Verification items for the finished model (mm, model axes). A direction names the side the tool comes from. Coordinates: 2 decimals unless noted, no trailing zeros. Order: outer loops, then holes, each group sorted by start corner. A loop starts at its lowest first (then second) coordinate and runs counter-clockwise, first axis right, second up.
Q1. Thickness scan on line 1 (Z direction, x = 0.75, y = 0.75); line 2 (X direction, y = 4.5, z = -1); line 3 (X direction, y = 3.75, z = 1.5). Record the ranges inside material, lowest first.
Q2. Cross-section at B-B, the plane y = 7.5. Record the boundary of the cut face in (x, z).
Q3. Set-up check for faces 1 (the flat face through (2, 11, 1.242)), 2 (the flat face through (-1.621, 10.034, -1.7)), 3 (the conical face through (-2.409, -2.189, 1.847)), 4 (the cylindrical face through (-0.9, 8.3, -2.1)), 5 (the conical face through (-1.913, 9.933, 0.04)): record each of +Z, -Z, +X, -X, +Y, -Y from which the full face is reachable in a straight line by a thin tool's end or side.
Q4. Draft check along Z on faces 6 (the flat face through (1.194, 9.5, 1.8)), 7 (the flat face through (-2, 11, -1.242)), 8 (the cylindrical face through (0.679, -2.129, -2.156)). Enter one of: pulls with the +Z half, pulls with the -Z half, needs draft (parallel to the pull), parting line crosses it, or undercut.
Q5. Cross-section at C-C, the plane y = 0.75. Record the boundary of the cut face in (x, z), and give its area (3 significant figures).
Q6. Depth check by flat-ended pin: P1, Ø1.5, axis at x = 0.5, z = 0.5, coming from the +Y side; P2, Ø0.7, axis at y = 9.5, z = 2, coming from the -X side; P3, Ø1, axis at x = 2, y = 11, coming from the +Z side. Enter the tip coordinate at first touch or a pass-through.
Q7. Cross-section at A-A, the plane y = -2. Record the boundary of the cut face in (x, z).
from build123d import *

# Parameters (mm, degrees)
SKETCH1_R                   = 2.9972
INSERT_DEPTH                = 11.811
INSERT_TAPER                = 2
INSERT_OTHER_WAY_DEPTH      = 4.318
INSERT_OTHER_WAY_TAPER      = -1
SKETCH2_R                   = 2.2606
INSERT_BORE_DEPTH           = 13.584955674
INSERT_BORE_TAPER           = 2
INSERT_BORE_OTHER_WAY_DEPTH = 13.584955674
PASS_CUT_DEPTH              = 13.584955674
PASS_CUT_DEPTH_BACK         = 13.584955674
PASS_CHIP_DEPTH             = 13.584955674
CIRPATTERN1_COUNT           = 2
SKETCH5_R                   = 2.032
BOSS_EXTRUDE1_DEPTH         = 1.0922


with BuildPart() as part:
    # Sketch1 → insert (new body)
    with BuildSketch(Plane(origin=(0, 0, 0), x_dir=(1, 0, 0), z_dir=(0, 1, 0))):
        Circle(SKETCH1_R)
    extrude(amount=INSERT_DEPTH, taper=INSERT_TAPER)

    # Sketch1 → insert other way (add)
    with BuildSketch(Plane(origin=(0, 0, 0), x_dir=(1, 0, 0), z_dir=(0, 1, 0))):
        Circle(SKETCH1_R)
    extrude(amount=-INSERT_OTHER_WAY_DEPTH, taper=INSERT_OTHER_WAY_TAPER)

    # Sketch2 → insert bore (cut)
    with BuildSketch(Plane.XZ):
        with Locations(Location((0, 0, 0), (0, 0, 270))):
            Circle(SKETCH2_R)
    extrude(amount=-INSERT_BORE_DEPTH, taper=INSERT_BORE_TAPER, mode=Mode.SUBTRACT)

    # Sketch2 → insert bore other way (cut)
    with BuildSketch(Plane.XZ):
        with Locations(Location((0, 0, 0), (0, 0, 270))):
            Circle(SKETCH2_R)
    extrude(amount=INSERT_BORE_OTHER_WAY_DEPTH, mode=Mode.SUBTRACT)

    # Sketch3 → pass cut (cut, two sides: drawn at the far end of the back side and taken through both)
    with BuildSketch(Plane.XY.offset(-PASS_CUT_DEPTH_BACK)):
        with BuildLine():
            Line((-1.1938, 11.811), (1.1938, 11.811))
            Line((1.1938, 11.811), (1.1938, 9.017))
            ThreePointArc((1.1938, 9.017), (0.89622049, 8.29857951), (0.1778, 8.001))
            Line((0.1778, 8.001), (-0.1778, 8.001))
            ThreePointArc((-0.1778, 8.001), (-0.89622049, 8.29857951), (-1.1938, 9.017))
            Line((-1.1938, 9.017), (-1.1938, 11.811))
        make_face()
    extrude(amount=PASS_CUT_DEPTH + PASS_CUT_DEPTH_BACK, mode=Mode.SUBTRACT)

    # Sketch4 → pass chip (cut, through all)
    with BuildSketch(Plane(origin=(0, 0, 0), x_dir=(0, 0, -1), z_dir=(1, 0, 0))):
        Polygon((1.242429972, 11.811), (2.707189518, 11.811), (2.707189518, 8.703141678), (1.242429972, 10.638716792), align=None)
    pass_chip = extrude(amount=-PASS_CHIP_DEPTH, mode=Mode.SUBTRACT)

    # CirPattern1: pass chip ×2 about axis
    cirpattern1_axis = Axis((0, -4.318, 0), (0, 1, 0))
    for i in range(1, CIRPATTERN1_COUNT):
        add(pass_chip.rotate(cirpattern1_axis, i * 360 / CIRPATTERN1_COUNT), mode=Mode.SUBTRACT)

    # Sketch5 → Boss-Extrude1 (add)
    with BuildSketch(Plane(origin=(0, 8.001, 0), x_dir=(-1, 0, 0), z_dir=(0, -1, 0))):
        Circle(SKETCH5_R)
    extrude(amount=BOSS_EXTRUDE1_DEPTH)


solid = part.part
Check values:
1. line 1: z = -2.87 to -2.1, 2.1 to 2.87
1. line 2: x = -2.66 to -1.85, 1.85 to 2.66
1. line 3: x = -2.44 to -1.51, 1.51 to 2.44
2. outline: circle Ø5.47 at (0, 0)
3. face 1: +Z, +X, +Y
3. face 2: -Z, -X, +Y
3. face 3: +Y
3. face 4: +Z, -Z, +Y
3. face 5: none
4. face 6: needs draft
4. face 7: pulls with the -Z half
4. face 8: undercut
5. outline: circle Ø5.94 at (0, 0); hole circle Ø4.47 at (0, 0)
5. area: 12.0 mm2
6. P1: stops at y = 8
6. P2: stops at x = -2.09
6. P3: stops at z = 1.35
7. outline: circle Ø6.06 at (0, 0); hole circle Ø4.52 at (0, 0)
